```python
from build123d import *

# Parameters (mm, degrees)
SKETCH1_W           = 203.2
SKETCH1_H           = 101.6
BOSS_EXTRUDE1_DEPTH = 5.08
SKETCH2_W           = 5.08
SKETCH2_H           = 25.4
SKETCH2_W_2         = 25.4
SKETCH2_H_2         = 5.08
CUT_EXTRUDE1_DEPTH  = 5.08


with BuildPart() as part:
    # Sketch1 → Boss-Extrude1 (new body)
    with BuildSketch(Plane.XY):
        with Locations((0, 50.8)):
            Rectangle(SKETCH1_W, SKETCH1_H)
        with Locations((0, -50.8)):
            Rectangle(SKETCH1_W, SKETCH1_H)
    extrude(amount=BOSS_EXTRUDE1_DEPTH)

    # Sketch2 → Cut-Extrude1 (cut)
    with BuildSketch(Plane(origin=(0, 0, 0), x_dir=(-1, 0, 0), z_dir=(0, 0, -1))):
        with Locations((-99.06, -44.45)):
            Rectangle(SKETCH2_W, SKETCH2_H)
        with Locations((99.06, -44.45)):
            Rectangle(SKETCH2_W, SKETCH2_H)
        with Locations((99.06, 63.5)):
            Rectangle(SKETCH2_W, SKETCH2_H)
        with Locations((46.99, 99.06)):
            Rectangle(SKETCH2_W_2, SKETCH2_H_2)
        with Locations((-46.99, 99.06)):
            Rectangle(SKETCH2_W_2, SKETCH2_H_2)
        with Locations((-99.06, 63.5)):
            Rectangle(SKETCH2_W, SKETCH2_H)
    extrude(amount=-CUT_EXTRUDE1_DEPTH, mode=Mode.SUBTRACT)


solid = part.part
```
Design review of the part built by this model. Coordinates are the model's own, in mm. A direction names the side the tool comes from. Give positions to 0.01 mm unless a question says otherwise; leave off trailing zeros. Loops run counter-clockwise (first coordinate to the right, second up) from the corner with the lowest first, then second, coordinate; pieces in that order, holes last. Notation, with made-up numbers: (35.25, 89) -> (66.25, 89) arc R20 cw to (66.25, 109) -> close; hole circle Ø1 at (3, -38.75). An arc over 180 degrees is marked (long way). One line per item, written item: value.
Q1. We need section B-B on y = 66.5. Give the boundary of the cut face in (x, z).
Numbers:
outline: (-96.52, 0) -> (96.52, 0) -> (96.52, 5.08) -> (-96.52, 5.08) -> close
Q2. We need section A-A on z = 3.8. Give the boundary of the cut face in (x, y).
Numbers:
outline: (-101.6, -101.6) -> (101.6, -101.6) -> (101.6, -57.15) -> (96.52, -57.15) -> (96.52, -31.75) -> (101.6, -31.75) -> (101.6, 50.8) -> (96.52, 50.8) -> (96.52, 76.2) -> (101.6, 76.2) -> (101.6, 101.6) -> (59.69, 101.6) -> (59.69, 96.52) -> (34.29, 96.52) -> (34.29, 101.6) -> (-34.29, 101.6) -> (-34.29, 96.52) -> (-59.69, 96.52) -> (-59.69, 101.6) -> (-101.6, 101.6) -> (-101.6, 76.2) -> (-96.52, 76.2) -> (-96.52, 50.8) -> (-101.6, 50.8) -> (-101.6, -31.75) -> (-96.52, -31.75) -> (-96.52, -57.15) -> (-101.6, -57.15) -> close
Q3. For L1, parallel to X at y = -49.5, z = 1.5; L2, parallel to Y at x = -57, z = 4, list the stretches that pass through material, from the lowest coordinate up.
Numbers:
L1: x = -96.52 to 96.52
L2: y = -101.6 to 96.52
Q4. Machinability: for faces 1 (the flat face through (-47, 96.52, 3)), 2 (the flat face through (101.6, 9, 3)), 3 (the flat face through (-96.52, 63, 3)), 4 (the flat face through (99, -57.15, 3)), 5 (the flat face through (0, 101.6, 3)), which of the approach directions +Z, -Z, +X, -X, +Y, -Y give a long, thin tool a straight path to every point of the face, cutting with its end or side? Answer none if there is none.
Numbers:
face 1: +Z, -Z, +Y
face 2: +Z, -Z, +X, +Y, -Y
face 3: +Z, -Z, -X
face 4: +Z, -Z, +X
face 5: +Z, -Z, +X, -X, +Y
Q5. Draft analysis for pull direction X (two halves, no side actions). For faces 6 (the flat face through (47, 96.52, 3)), 7 (the flat face through (-101.6, 89, 3)), 8 (the flat face through (-1, 1, 0)), state which applies: pulls with the +X half, pulls with the -X half, needs draft (parallel to the pull), parting line crosses it, or undercut.
Numbers:
face 6: undercut
face 7: pulls with the -X half
face 8: needs draft
Q6. For pin 1 Ø2.5 at (x, z) = (45, 2) entering from +Y; pin 2 Ø1.5 at (y, z) = (-48.5, 2) entering from -X, all flat-tipped, find the tip position at first contact; note any pin that passes through.
Numbers:
pin 1: stops at y = 96.52
pin 2: stops at x = -96.52
